Work out the finished part from the listing and answer in its coordinate system (mm). A direction names the side the tool comes from. Coordinates: 2 decimals unless noted, no trailing zeros. Order: outer loops, then holes, each group sorted by start corner. A loop starts at its lowest first (then second) coordinate and runs counter-clockwise, first axis right, second up. Notation, with made-up numbers: (67, 55.25) - (116, 55.25) arc R16 ccw to (116, 68.25) - close; hole circle Ø2 at (-26.5, -23.5). An arc over 180 degrees is marked (long way). Answer as a JSON object with one key per item and string values. Group by question number.
1) Section D-D (x = 18) is taken. Give the vertices of the cut face in (y, z), plus the area to 3 significant figures.
2) Find the intervals of material crossed by line 1 along X through (y, z) = (24.75, 40.6); line 2 along Y through (x, z) = (6, 40.65); line 3 along Y through (x, z) = (21.5, 41.7), in increasing order.
3) Section C-C (z = 40.65) is taken. Give the vertices of the cut face in (x, y).
4) Each of these flat-tipped pins is pushed along its axis until it touches: P1, Ø0.5, axis at x = 9, z = 40.5, coming from the +Y side; P2, Ø0.8, axis at y = 20.5, z = 40.5, coming from the -X side; P3, Ø0.5, axis at y = 25.5, z = 40.5, coming from the +X side. Where does it stop, or does it pass through?
5) A tool of negligible diameter and unlimited length cuts with its end or side. For faces 1 (the face through (18.3, 37.703, 40.5)), 2 (the face through (-3.887, 25.5, 40.5)), 3 (the face through (41.113, 25.5, 40.5)), from which of +Z, -Z, +X, -X, +Y, -Y can it reach the whole face along a straight path? Write none if from no direction.
6) Section B-B (x = 1) is taken. Give the vertices of the cut face in (y, z).
7) Section A-A (y = 27.5) is taken. Give the vertices of the cut face in (x, z), plus the area to 3 significant figures.
from build123d import *

# Parameters (mm, degrees)
BOSS_EXTRUDE1_DEPTH = 1
SKETCH2_W           = 45
SKETCH2_H           = 24
BOSS_EXTRUDE2_DEPTH = 2


with BuildPart() as part:
    # Sketch1 → Boss-Extrude1 (new body)
    with BuildSketch(Plane.XY.offset(40.959042005)):
        Polygon((41.113098235, 13.703029386), (21.556960057, 13.703029386), (21.556960057, 12.703029386), (42.113098235, 12.703029386), (42.113098235, 38.703029386), (-4.886901765, 38.703029386), (-4.886901765, 12.703029386), (16.495104543, 12.703029386), (16.495104543, 13.703029386), (-3.886901765, 13.703029386), (-3.886901765, 37.703029386), (41.113098235, 37.703029386), align=None)
    extrude(amount=BOSS_EXTRUDE1_DEPTH)

    # Sketch2 → Boss-Extrude2 (add)
    with BuildSketch(Plane.XY.offset(41.959042005)):
        with Locations((18.613098235, 25.703029386)):
            Rectangle(SKETCH2_W, SKETCH2_H)
    extrude(amount=-BOSS_EXTRUDE2_DEPTH)


solid = part.part
Report:
{
 "1": {"outline": "(13.7, 39.96) - (37.7, 39.96) - (37.7, 40.96) - (38.7, 40.96) - (38.7, 41.96) - (13.7, 41.96) - close", "area": "49.0 mm²"},
 "2": {"line 1": "x = -3.89 to 41.11", "line 2": "y = 13.7 to 37.7", "line 3": "y = 13.7 to 38.7"},
 "3": {"outline": "(-3.89, 13.7) - (41.11, 13.7) - (41.11, 37.7) - (-3.89, 37.7) - close"},
 "4": {"P1": "stops at y = 37.7", "P2": "stops at x = -3.89", "P3": "stops at x = 41.11"},
 "5": {"face 1": "-Z, +X, -X, +Y", "face 2": "-Z, -X, +Y, -Y", "face 3": "-Z, +X, +Y, -Y"},
 "6": {"outline": "(12.7, 40.96) - (13.7, 40.96) - (13.7, 39.96) - (37.7, 39.96) - (37.7, 40.96) - (38.7, 40.96) - (38.7, 41.96) - (12.7, 41.96) - close"},
 "7": {"outline": "(-4.89, 40.96) - (-3.89, 40.96) - (-3.89, 39.96) - (41.11, 39.96) - (41.11, 40.96) - (42.11, 40.96) - (42.11, 41.96) - (-4.89, 41.96) - close", "area": "92.0 mm²"}
}
